Input: part model. Units: mm. Frame: model coordinates. A direction names the side the tool comes from. Round coordinates to 2 decimals unless told otherwise and drop trailing zeros. Loops run counter-clockwise (first coordinate to the right, second up) from the corner with the lowest first, then second, coordinate; pieces in that order, holes last. Notation, with made-up numbers: (87, 33) -> (110, 33) arc R24 ccw to (110, 54) -> close; hole circle Ø10 at (-28, 11). An arc over 180 degrees is marked (long way). One line per question, with ' | ' between items. Start each with the question number.
Q1. Cut plane A-A on x = 0. Return loops of the section in (y, z).
Q2. Cut plane B-B on z = 0.7. Return loops of the section in (x, y), and give its area (3 significant figures).
Q3. Access query for faces 5 (the face through (-33.91, -36.068, 0.789)), 6 (the face through (-12.196, -21.789, 0.811)). Directions: +Z, -Z, +X, -X, +Y, -Y. A direction counts if a zero-diameter tool reaches every point of the face in a straight line with its end or side. Return the directions, or none.
Q4. Material intervals for L1, parallel to X at y = -34.5, z = 1.3; L2, parallel to X at y = 1.5, z = 0.95; L3, parallel to Y at x = 34, z = 0.9, sorted ascending.
Q5. Cut plane D-D on y = 0. Return loops of the section in (x, z).
Q6. Contact query for flat-ended pins moving along their axis: P1, Ø0.8, axis at y = -3.5, z = 0.5, coming from the +X side; P2, Ø0.5, axis at x = 29.5, z = 1, coming from the -Y side. Output: stop coordinate, or through.
Q7. Cut plane C-C on x = 14. Return loops of the section in (y, z), and give its area (3 significant figures).
Q8. Mould query, pull axis Y, two halves, no side actions, for faces 1 (the face through (-12.289, 21.696, 0.811)), 2 (the face through (47.369, 25.053, 0.811)), 3 (the face through (-54.963, 2.007, 0.789)), 4 (the face through (-16, 1, 1.6)). Classes: pulls with the +Y half, pulls with the -Y half, needs draft (parallel to the pull), parting line crosses it, or undercut.
from build123d import *

# Parameters (mm, degrees)
SKETCH_1_R      = 1.6
EXTRUDE_1_DEPTH = 1.6
FILLET_1_R      = 6
FILLET_2_R      = 3


with BuildPart() as part:
    # 草圖1 → 填料-伸長1 (new body)
    with BuildSketch(Plane.XY):
        with BuildLine():
            Line((49.726753363, -23.5), (-14, -23.5))
            Line((-14, -23.5), (-14, 23.5))
            Line((-14, 23.5), (49.726753363, 23.5))
            ThreePointArc((49.726753363, 23.5), (-55, 0), (49.726753363, -23.5))
        make_face()
        with Locations((34.648232278, 34.648232278)):
            Circle(SKETCH_1_R, mode=Mode.SUBTRACT)
        with Locations((-34.648232278, 34.648232278)):
            Circle(SKETCH_1_R, mode=Mode.SUBTRACT)
        with Locations((-34.648232278, -34.648232278)):
            Circle(SKETCH_1_R, mode=Mode.SUBTRACT)
        with Locations((34.648232278, -34.648232278)):
            Circle(SKETCH_1_R, mode=Mode.SUBTRACT)
    extrude(amount=EXTRUDE_1_DEPTH)

    # 圓角1
    fillet_1_edges = [part.edges().sort_by_distance(p)[0] for p in [
        (-14, 23.5, 0.8),
        (-14, -23.5, 0.8),
    ]]
    fillet(fillet_1_edges, radius=FILLET_1_R)

    # 圓角2
    fillet_2_edges = [part.edges().sort_by_distance(p)[0] for p in [
        (49.726753363, 23.5, 0.8),
        (49.726753363, -23.5, 0.8),
    ]]
    fillet(fillet_2_edges, radius=FILLET_2_R)


solid = part.part
Results:
1) outline: (-55, 0) -> (-23.5, 0) -> (-23.5, 1.6) -> (-55, 1.6) -> close; (23.5, 0) -> (55, 0) -> (55, 1.6) -> (23.5, 1.6) -> close
2) outline: (-14, -17.5) -> (-14, 17.5) arc R6 cw to (-8, 23.5) -> (44.74, 23.5) arc R3 ccw to (47.32, 28.03) arc R55 ccw (long way) to (47.32, -28.03) arc R3 ccw to (44.74, -23.5) -> (-8, -23.5) arc R6 cw to start; hole circle Ø3.2 at (-34.65, -34.65); hole circle Ø3.2 at (-34.65, 34.65); hole circle Ø3.2 at (34.65, -34.65); hole circle Ø3.2 at (34.65, 34.65) | area: 6,310 mm^2
3) face 5: +Z, -Z | face 6: +Z, -Z, +X
4) L1: -42.83 to -36.24, -33.06 to 33.06, 36.24 to 42.83 | L2: -54.98 to -14 | L3: -43.23 to -36.11, -33.19 to -23.5, 23.5 to 33.19, 36.11 to 43.23
5) outline: (-55, 0) -> (-14, 0) -> (-14, 1.6) -> (-55, 1.6) -> close
6) P1: x = -14 | P2: y = -46.58
7) outline: (-53.19, 0) -> (-23.5, 0) -> (-23.5, 1.6) -> (-53.19, 1.6) -> close; (23.5, 0) -> (53.19, 0) -> (53.19, 1.6) -> (23.5, 1.6) -> close | area: 95.0 mm^2
8) face 1: undercut | face 2: undercut | face 3: parting line crosses it | face 4: needs draft
